Build history of the part. All positions in model axes, mm. A direction names the side the tool comes from. Give positions to 0.01 mm unless a question says otherwise; leave off trailing zeros. Loops run counter-clockwise (first coordinate to the right, second up) from the corner with the lowest first, then second, coordinate; pieces in that order, holes last. Notation, with made-up numbers: M -6,28.25 L 43,28.25 A26 cw 43,48.25 Z; hole C 5,20.25 d2. An arc over 180 degrees is marked long. Answer as a JSON object with one key per item and string values. Group by question number.
1. Drill centre lines: line 1 along X through (y, z) = (48.95, -91.25); line 2 along X through (y, z) = (-48.75, 0); line 3 along Z through (x, y) = (86, -48). Where is each one in solid material? Low to high. Write a range as [from, to].
2. Mould opens along Z. For faces 1 (the face through (-89.18, -48.48, -0.65)), 2 (the face through (-80, -47, -8)), 3 (the face through (0.132, 48.521, 88.253)), 4 (the face through (-1, 1, 82.5)) say: released by +Z, released by -Z, zero draft, split by the parting line, or undercut.
3. Slice it at A-A (z = 91.25). Give the number of separate pieces and of enclosed holes in the cut face, then the cut area to 3 significant figures.
4. Slice it at B-B (x = 67.5). List the corners of the cut face in (y, z).
5. 3-axis set-ups, long thin cutter, end or side, ignore diameter. For faces 5 (the face through (-1, 1, -80)), 6 (the face through (77, 5, 45)), 7 (the face through (77.5, 1, 1)): which of +Z, -Z, +X, -X, +Y, -Y reach the whole face in a straight line?
6. Drop flat-ended pins along their axis: pin 1 Ø5 at (x, z) = (-86.25, -91.25) entering from -Y; pin 2 Ø4 at (x, y) = (-50, 4.5) entering from +Z; pin 3 Ø1.5 at (y, z) = (-36.5, 5.5) entering from -X; pin 4 Ø7 at (x, z) = (0, -91.25) entering from -Y. Give the stop position or say it passes through.
from build123d import *

# Parameters (mm, degrees)
SKETCH1_W           = 155
SKETCH1_H           = 165
SKETCH1_W_2         = 150
SKETCH1_H_2         = 160
BOSS_EXTRUDE1_DEPTH = 50
SKETCH2_W           = 26
SKETCH2_H           = 36
CUT_EXTRUDE1_DEPTH  = 183.568480303
CUT_EXTRUDE2_START  = -2
SKETCH3_W           = 46
SKETCH3_H           = 56
CUT_EXTRUDE2_DEPTH  = 154
SKETCH4_W           = 195
SKETCH4_H           = 205
SKETCH4_W_2         = 155
SKETCH4_H_2         = 165
BOSS_EXTRUDE2_DEPTH = 3
BOSS_EXTRUDE3_START = -100
SKETCH4_2_W         = 195
SKETCH4_2_H         = 205
SKETCH4_2_W_2       = 155
SKETCH4_2_H_2       = 165
BOSS_EXTRUDE3_DEPTH = 3
SKETCH5_R           = 3
CUT_EXTRUDE3_DEPTH  = 174.241161391


with BuildPart() as part:
    # Sketch1 → Boss-Extrude1 (new, symmetric)
    with BuildSketch(Plane(origin=(0, 0, 0), x_dir=(1, 0, 0), z_dir=(0, 1, 0))):
        Rectangle(SKETCH1_W, SKETCH1_H)
        Rectangle(SKETCH1_W_2, SKETCH1_H_2, mode=Mode.SUBTRACT)
    extrude(amount=BOSS_EXTRUDE1_DEPTH, both=True)

    # Sketch2 → Cut-Extrude1 (cut, through all)
    with BuildSketch(Plane(origin=(77.5, 0, 0), x_dir=(0, 0, -1), z_dir=(1, 0, 0))):
        with Locations((-30, 5)):
            Rectangle(SKETCH2_W, SKETCH2_H)
        with Locations((30, 5)):
            Rectangle(SKETCH2_W, SKETCH2_H)
    extrude(amount=-CUT_EXTRUDE1_DEPTH, mode=Mode.SUBTRACT)

    # Sketch3 → Cut-Extrude2 (cut)
    with BuildSketch(Plane.ZY.offset(-75).offset(CUT_EXTRUDE2_START)):
        with Locations((-30, 5)):
            Rectangle(SKETCH3_W, SKETCH3_H)
        with Locations((30, 5)):
            Rectangle(SKETCH3_W, SKETCH3_H)
    extrude(amount=CUT_EXTRUDE2_DEPTH, mode=Mode.SUBTRACT)

    # Sketch4 → Boss-Extrude2 (add)
    with BuildSketch(Plane(origin=(0, 50, 0), x_dir=(1, 0, 0), z_dir=(0, 1, 0))):
        Rectangle(SKETCH4_W, SKETCH4_H)
        Rectangle(SKETCH4_W_2, SKETCH4_H_2, mode=Mode.SUBTRACT)
    extrude(amount=-BOSS_EXTRUDE2_DEPTH)

    # Sketch4<2> → Boss-Extrude3 (add)
    with BuildSketch(Plane(origin=(0, 50, 0), x_dir=(1, 0, 0), z_dir=(0, 1, 0)).offset(BOSS_EXTRUDE3_START)):
        Rectangle(SKETCH4_2_W, SKETCH4_2_H)
        Rectangle(SKETCH4_2_W_2, SKETCH4_2_H_2, mode=Mode.SUBTRACT)
    extrude(amount=BOSS_EXTRUDE3_DEPTH)

    # Sketch5 → Cut-Extrude3 (cut, through all)
    with BuildSketch(Plane(origin=(0, 50, 0), x_dir=(1, 0, 0), z_dir=(0, 1, 0))):
        with Locations(Location((-86.25, 91.25, 0), (0, 0, 270))):
            Circle(SKETCH5_R)
        with Locations(Location((0, 91.25, 0), (0, 0, 270))):
            Circle(SKETCH5_R)
        with Locations(Location((86.25, 91.25, 0), (0, 0, 270))):
            Circle(SKETCH5_R)
        with Locations(Location((-86.25, 0, 0), (0, 0, 270))):
            Circle(SKETCH5_R)
        with Locations(Location((86.25, 0, 0), (0, 0, 270))):
            Circle(SKETCH5_R)
        with Locations(Location((86.25, -91.25, 0), (0, 0, 270))):
            Circle(SKETCH5_R)
        with Locations(Location((0, -91.25, 0), (0, 0, 270))):
            Circle(SKETCH5_R)
        with Locations(Location((-86.25, -91.25, 0), (0, 0, 270))):
            Circle(SKETCH5_R)
    extrude(amount=-CUT_EXTRUDE3_DEPTH, mode=Mode.SUBTRACT)


solid = part.part
Established:
{
 "1": {"line 1": "x = [-97.5, -89.25], [-83.25, -3], [3, 83.25], [89.25, 97.5]", "line 2": "x = [-97.5, -89.25], [-83.25, -75], [75, 83.25], [89.25, 97.5]", "line 3": "z = [-102.5, -94.24], [-88.26, -2.99], [2.99, 88.26], [94.24, 102.5]"},
 "2": {"face 1": "undercut", "face 2": "zero draft", "face 3": "undercut", "face 4": "released by +Z"},
 "3": {"separate pieces": "8", "enclosed holes": "0", "area": "1,060 mm^2"},
 "4": {"outline": "M -50,-102.5 L -47,-102.5 L -47,-82.5 L 47,-82.5 L 47,-102.5 L 50,-102.5 L 50,-80 L -50,-80 Z; M -50,80 L 50,80 L 50,102.5 L 47,102.5 L 47,82.5 L -47,82.5 L -47,102.5 L -50,102.5 Z"},
 "5": {"face 5": "+Y, -Y", "face 6": "none", "face 7": "+Z, -Z, +X"},
 "6": {"pin 1": "passes through", "pin 2": "stops at z = 82.5", "pin 3": "stops at x = -77.5", "pin 4": "stops at y = -50"}
}
